from build123d import *

# Parameters (mm, degrees)
F1_DEPTH = 127
F2_R     = 38.7298959395
F3_DEPTH = 127
F4_DEPTH = 127
F5_DEPTH = 127
F7_DEPTH = 50.8
F9_DEPTH = 50.8


with BuildPart() as f1:
    # F0 (on Front) → F1 (new body)
    with BuildSketch(Plane.XZ):
        Polygon((-163.7962559972, -23.8678936321), (-163.4352315129, 77.7321063679), (-239.6352315129, 77.7321063679), (-239.6352315129, -74.6678936321), (-112.6352315129, -74.6678936321), (-130.5957437551, -56.70738139), (-54.3957437551, -56.70738139), (-72.3562559972, -74.6678936321), (-21.5562559972, -74.6678936321), (-21.5562559972, -23.8678936321), align=None)
    extrude(amount=F1_DEPTH)

    # F2 (on Top) → F3 (cut)
    with BuildSketch(Plane.XY):
        with Locations((-233.6748705878, -64.917108044)):
            Circle(F2_R)
    extrude(amount=F3_DEPTH, mode=Mode.SUBTRACT)

    # F4 (cut): a face of the model
    f4_faces = [f1.faces().sort_by_distance(p)[0] for p in [
        (-220.4073030245, -64.917108044, 0),
    ]]
    extrude(f4_faces, amount=-F4_DEPTH, mode=Mode.SUBTRACT)

    # F0 (on Front) → F5 (join)
    with BuildSketch(Plane.XZ):
        Polygon((-21.5562559972, -23.8678936321), (-163.4352315129, 77.7321063679), (-163.7962559972, -23.8678936321), align=None)
    extrude(amount=F5_DEPTH)

    # F6 (on face) → F7 (cut)
    with BuildSketch(Plane.XZ.offset(127)):
        Polygon((-21.5562559972, -23.8678936321), (-163.4352315129, 77.7321063679), (-163.4352315129, -23.8678936321), align=None)
    extrude(amount=-F7_DEPTH, mode=Mode.SUBTRACT)

    # F8 (on face) → F9 (cut)
    with BuildSketch(Plane.XZ):
        Polygon((-162.8829091787, -23.5076323152), (-20.4247385263, -23.5076323152), (-162.8829091787, 78.0534595251), align=None)
    extrude(amount=F9_DEPTH, mode=Mode.SUBTRACT)


solid = f1.part
Here's how the part is built. I have some questions about the finished solid (model axes, mm). A direction names the side the tool comes from. Coordinates: 2 decimals unless noted, no trailing zeros. Order: outer loops, then holes, each group sorted by start corner. A loop starts at its lowest first (then second) coordinate and runs counter-clockwise, first axis right, second up. Notation, with made-up numbers: (5.5, 61.5) -> (37.5, 61.5) arc R29 cw to (37.5, 85.5) -> close; hole circle Ø3 at (75, -31.75). An arc over 180 degrees is marked (long way). Answer in a Markdown table with one row per item.
(1) Will these pins go through, and if not, where does the flat tip stop? pin 1 Ø3 at (y, z) = (-39.5, 53.5) entering from -X; pin 2 Ø5 at (x, z) = (-47, -13.5) entering from +Y; pin 3 Ø2 at (y, z) = (-45.5, 48.5) entering from -X.
Answer key:
| item | result |
|---|---|
| pin 1 | x = -205.83 |
| pin 2 | y = -50.8 |
| pin 3 | x = -200.76 |
(2) On a 3-axis mill with a long thin cutter (end or side, diameter ignored), from which of +Z, -Z, +X, -X, +Y, -Y can I reach the whole of each face in a straight line? I mean faces 1 (the face through (-163, -63, -74.668)), 2 (the face through (-125, -76.2, 5)), 3 (the face through (-121.49, -62.611, -65.813)), 4 (the face through (-239.635, -115, 3)), 5 (the face through (-93, -25, -23.508)). Say none if no direction works.
Answer key:
| item | result |
|---|---|
| face 1 | -Z, +X, -X, +Y, -Y |
| face 2 | +Z, +X, -Y |
| face 3 | +Y, -Y |
| face 4 | +Z, -Z, -X, +Y, -Y |
| face 5 | +Z, +X, +Y |
(3) I want a section at D-D on x = -146. List the corners of the cut face in (y, z) for me.
Answer key:
| item | result |
|---|---|
| outline | (-127, -74.67) -> (0, -74.67) -> (0, -23.51) -> (-50.8, -23.51) -> (-50.8, 65.25) -> (-76.2, 65.25) -> (-76.2, -23.87) -> (-127, -23.87) -> close |
(4) Please list where these lines run through material, in increasing order: probe 1 along Y at (x, z) = (-72, -22); probe 2 along X at (y, z) = (-94.5, -61.5); probe 3 along Z at (x, y) = (-121, -45.5).
Answer key:
| item | result |
|---|---|
| probe 1 | -76.2 to -50.8 |
| probe 2 | -208.68 to -125.8, -59.19 to -21.56 |
| probe 3 | -74.67 to -66.3, -56.71 to -23.51 |
(5) I want a section at B-B on x = -66.5. List the corners of the cut face in (y, z) for me.
Answer key:
| item | result |
|---|---|
| outline | (-127, -74.67) -> (0, -74.67) -> (0, -68.81) -> (-127, -68.81) -> close; (-127, -56.71) -> (0, -56.71) -> (0, -23.51) -> (-50.8, -23.51) -> (-50.8, 8.32) -> (-76.2, 8.32) -> (-76.2, -23.87) -> (-127, -23.87) -> close |
(6) I want a section at A-A on y = -109. List the corners of the cut face in (x, z) for me, then the cut area to 3 significant figures.
Answer key:
| item | result |
|---|---|
| outline | (-239.64, -74.67) -> (-112.64, -74.67) -> (-130.6, -56.71) -> (-54.4, -56.71) -> (-72.36, -74.67) -> (-21.56, -74.67) -> (-21.56, -23.87) -> (-163.44, -23.87) -> (-163.44, 77.73) -> (-239.64, 77.73) -> close |
| area | 17,800 mm^2 |
(7) Thinking about a two-plate mould opening in Y: for faces 6 (the face through (-125, -50.8, 5)), 7 (the face through (-194.956, -65.853, 0.465)), 8 (the face through (-92.165, -60.5, 26.695)), which applies, +Y half, -Y half, draft (parallel to the pull), parting line (faces both ways), or undercut?
Answer key:
| item | result |
|---|---|
| face 6 | +Y half |
| face 7 | undercut |
| face 8 | draft |
(8) I want a section at C-C on z = -64.5. List the corners of the cut face in (x, y) for me.
Answer key:
| item | result |
|---|---|
| outline | (-239.64, -127) -> (-122.8, -127) -> (-122.8, 0) -> (-239.64, 0) -> (-239.64, -26.65) arc R38.73 cw (long way) to (-239.64, -103.19) -> close; (-62.19, -127) -> (-21.56, -127) -> (-21.56, 0) -> (-62.19, 0) -> close |
